Read the model definition and answer for the solid it produces. Units are mm, in the model's axes. A direction names the side the tool comes from. Round coordinates to 2 decimals unless told otherwise and drop trailing zeros. Write each question's results on one line, items separated by ' | '.
from build123d import *

# Parameters (mm, degrees)
F0_R     = 50.8
F0_R_2   = 44.45
F1_DEPTH = 6.35
F2_DEPTH = 10
F7_DEPTH = 88.9
F9_DEPTH = 88.9


# Not quite as in the source:
# - a fillet or chamfer that OpenCascade refuses, or shapes differently, is made with other operations: its cross-section is extruded or revolved along the edge and cut away or added


with BuildPart() as f1:
    # F0 (on Top) → F1 (new body)
    with BuildSketch(Plane.XY):
        Circle(F0_R)
        Circle(F0_R_2, mode=Mode.SUBTRACT)
    extrude(amount=F1_DEPTH)

    # F0 (on Top) → F2 (join)
    with BuildSketch(Plane.XY):
        Circle(F0_R_2)
    extrude(amount=F2_DEPTH)

    # F6 (on face) → F7 (cut)
    with BuildSketch(Plane(origin=(0, -44.45, 0), x_dir=(-1, 0, 0), z_dir=(0, 1, 0))):
        Polygon((39.45, 6.35), (44.45, 10), (34.45, 10), align=None)
        Polygon((29.45, 6.35), (34.45, 10), (24.45, 10), align=None)
        Polygon((19.4500000001, 6.35), (24.45, 10), (14.4500000001, 10), align=None)
        Polygon((9.4500000001, 6.35), (14.4500000001, 10), (4.4500000002, 10), align=None)
        Polygon((-0.5499999998, 6.35), (4.4500000002, 10), (-5.5499999998, 10), align=None)
        Polygon((-10.5499999998, 6.35), (-5.5499999998, 10), (-15.5499999998, 10), align=None)
        Polygon((-20.5499999997, 6.35), (-15.5499999998, 10), (-25.5499999997, 10), align=None)
        Polygon((-30.5499999997, 6.35), (-25.5499999997, 10), (-35.5499999997, 10), align=None)
        Polygon((-40.5499999997, 6.35), (-35.5499999997, 10), (-45.5499999996, 10), align=None)
    extrude(amount=F7_DEPTH, mode=Mode.SUBTRACT)

    # F8 (on face) → F9 (cut)
    with BuildSketch(Plane(origin=(22.225, -38.4948291982, 0), x_dir=(0.8660254038, 0.5, 0), z_dir=(0.5, -0.8660254038, 0))):
        Polygon((-33.8791470656, 10), (-43.8791470656, 10), (-38.8791470656, 6.35), align=None)
        Polygon((-23.8791470657, 10), (-33.8791470656, 10), (-28.8791470656, 6.35), align=None)
        Polygon((-13.8791470657, 10), (-23.8791470657, 10), (-18.8791470657, 6.35), align=None)
        Polygon((-3.8791470657, 10), (-13.8791470657, 10), (-8.8791470657, 6.35), align=None)
        Polygon((6.1208529342, 10), (-3.8791470657, 10), (1.1208529342, 6.35), align=None)
        Polygon((16.1208529342, 10), (6.1208529342, 10), (11.1208529342, 6.35), align=None)
        Polygon((26.1208529341, 10), (16.1208529342, 10), (21.1208529342, 6.35), align=None)
        Polygon((36.1208529341, 10), (26.1208529341, 10), (31.1208529341, 6.35), align=None)
        Polygon((46.1208529341, 10), (36.1208529341, 10), (41.1208529341, 6.35), align=None)
    extrude(amount=-F9_DEPTH, mode=Mode.SUBTRACT)

    # F10: fillet of radius 2.54 on 1 edges, made by hand

    # F10_s1 → F10_t2 (revolve, cut)
    with BuildSketch(Plane.XZ):
        with BuildLine():
            ThreePointArc((50.8, 3.81), (50.0560512242, 5.6060512242), (48.26, 6.35))
            Line((48.26, 6.35), (50.8, 6.35))
            Line((50.8, 6.35), (50.8, 3.81))
        make_face()
    revolve(axis=Axis((0, 0, 6.35), (0, 0, -1)), mode=Mode.SUBTRACT)


solid = f1.part
Item 1: Straight lines are drawn through the part: line 1 (Z direction, x = -46, y = -7); line 2 (Z direction, x = -41.5, y = -0.5); line 3 (X direction, y = -37.5, z = 1). For each, find the intervals that lie inside material, in ascending order.
Outcome:
line 1: z = 0 to 6.35 | line 2: z = 0 to 7.85 | line 3: x = -34.27 to 34.27
Item 2: For faces 1 (the face through (42.767, 12.115, 6.932)), 2 (the face through (21.974, 14.286, 7.389)), 3 (the face through (-3.837, -27.293, 7.744)), determine the directions among +Z, -Z, +X, -X, +Y, -Y from which every point of the face is accessible in a straight line to the end or side of a thin tool.
Outcome:
face 1: +Z, +X, +Y | face 2: +Z, +Y, -Y | face 3: +Z
Item 3: The mould has two halves that part along X. Classify faces 4 (the face through (-8.026, 6.247, 7.389)), 5 (the face through (-15.681, 41.592, 7.419)), 6 (the face through (42.035, -14.453, 6.671)): pulls with the +X half, pulls with the -X half, needs draft (parallel to the pull), parting line crosses it, or undercut.
Outcome:
face 4: undercut | face 5: pulls with the -X half | face 6: pulls with the +X half
Item 4: Flat-ended cylindrical pins translate along their axes: pin 1 (4 mm diameter, centred on x = 4.5, z = 6.5, fed in from +Y); pin 2 (2 mm diameter, centred on x = 38.5, y = 22.5, fed in from +Z); pin 3 (1.5 mm diameter, centred on y = -6, z = 5, fed in from -X). Find the tip coordinate at first contact, or state that the pin passes through.
Outcome:
pin 1: stops at y = 50.53 | pin 2: stops at z = 8.49 | pin 3: stops at x = -50.43
